from build123d import *

# Parameters (mm, degrees)
SKETCH_R     = 1
SKETCH_W     = 14
SKETCH_H     = 14
PAD_DEPTH    = 1.5
POCKET_START = 1
SKETCH001_R  = 2
POCKET_DEPTH = 14


with BuildPart() as part:
    # Sketch → Pad (new body)
    with BuildSketch(Plane.XY):
        with BuildLine():
            Line((115.15, 33), (115.15, 110.15))
            ThreePointArc((115.15, 110.15), (113.685534, 113.685534), (110.15, 115.15))
            Line((110.15, 115.15), (11, 115.15))
            ThreePointArc((11, 115.15), (7.464466, 113.685534), (6, 110.15))
            Line((6, 110.15), (6, 33))
            ThreePointArc((6, 33), (7.464466, 29.464466), (11, 28))
            Line((11, 28), (110.15, 28))
            ThreePointArc((110.15, 28), (113.685534, 29.464466), (115.15, 33))
        make_face()
        with Locations((10, 111.15)):
            Circle(SKETCH_R, mode=Mode.SUBTRACT)
        with Locations((10, 32)):
            Circle(SKETCH_R, mode=Mode.SUBTRACT)
        with Locations((111.15, 32)):
            Circle(SKETCH_R, mode=Mode.SUBTRACT)
        with Locations((111.15, 111.15)):
            Circle(SKETCH_R, mode=Mode.SUBTRACT)
        with Locations((71.55, 71.55)):
            Circle(SKETCH_R, mode=Mode.SUBTRACT)
        with Locations((33.5, 71.55)):
            Circle(SKETCH_R, mode=Mode.SUBTRACT)
        with Locations((31.5, 62.05)):
            Circle(SKETCH_R, mode=Mode.SUBTRACT)
        with Locations((10, 62.05)):
            Circle(SKETCH_R, mode=Mode.SUBTRACT)
        with Locations((10, 40.55)):
            Circle(SKETCH_R, mode=Mode.SUBTRACT)
        with Locations((31.5, 40.55)):
            Circle(SKETCH_R, mode=Mode.SUBTRACT)
        with Locations((43, 43)):
            Rectangle(SKETCH_W, SKETCH_H, mode=Mode.SUBTRACT)
        with Locations((62.05, 43)):
            Rectangle(SKETCH_W, SKETCH_H, mode=Mode.SUBTRACT)
        with Locations((81.1, 43)):
            Rectangle(SKETCH_W, SKETCH_H, mode=Mode.SUBTRACT)
        with Locations((100.15, 43)):
            Rectangle(SKETCH_W, SKETCH_H, mode=Mode.SUBTRACT)
        with Locations((43, 62.05)):
            Rectangle(SKETCH_W, SKETCH_H, mode=Mode.SUBTRACT)
        with Locations((62.05, 62.05)):
            Rectangle(SKETCH_W, SKETCH_H, mode=Mode.SUBTRACT)
        with Locations((81.1, 62.05)):
            Rectangle(SKETCH_W, SKETCH_H, mode=Mode.SUBTRACT)
        with Locations((100.15, 62.05)):
            Rectangle(SKETCH_W, SKETCH_H, mode=Mode.SUBTRACT)
        with Locations((43, 81.1)):
            Rectangle(SKETCH_W, SKETCH_H, mode=Mode.SUBTRACT)
        with Locations((62.05, 81.1)):
            Rectangle(SKETCH_W, SKETCH_H, mode=Mode.SUBTRACT)
        with Locations((81.1, 81.1)):
            Rectangle(SKETCH_W, SKETCH_H, mode=Mode.SUBTRACT)
        with Locations((100.15, 81.1)):
            Rectangle(SKETCH_W, SKETCH_H, mode=Mode.SUBTRACT)
        with Locations((43, 100.15)):
            Rectangle(SKETCH_W, SKETCH_H, mode=Mode.SUBTRACT)
        with Locations((62.05, 100.15)):
            Rectangle(SKETCH_W, SKETCH_H, mode=Mode.SUBTRACT)
        with Locations((81.1, 100.15)):
            Rectangle(SKETCH_W, SKETCH_H, mode=Mode.SUBTRACT)
        with Locations((100.15, 100.15)):
            Rectangle(SKETCH_W, SKETCH_H, mode=Mode.SUBTRACT)
        with BuildLine():
            ThreePointArc((16.25, 111.15), (15, 112.4), (13.75, 111.15))
            Line((13.75, 111.15), (13.75, 79.15))
            ThreePointArc((13.75, 79.15), (15, 77.9), (16.25, 79.15))
            Line((16.25, 111.15), (16.25, 79.15))
        make_face(mode=Mode.SUBTRACT)
        with BuildLine():
            ThreePointArc((31.25, 111.15), (30, 112.4), (28.75, 111.15))
            Line((28.75, 111.15), (28.75, 79.15))
            ThreePointArc((28.75, 79.15), (30, 77.9), (31.25, 79.15))
            Line((31.25, 111.15), (31.25, 79.15))
        make_face(mode=Mode.SUBTRACT)
        with BuildLine():
            ThreePointArc((15.75, 63.05), (14.75, 62.05), (15.75, 61.05))
            Line((15.75, 61.05), (25.75, 61.05))
            ThreePointArc((25.75, 61.05), (26.75, 62.05), (25.75, 63.05))
            Line((15.75, 63.05), (25.75, 63.05))
        make_face(mode=Mode.SUBTRACT)
    extrude(amount=PAD_DEPTH)

    # Sketch001 → Pocket (cut)
    with BuildSketch(Plane.XY.offset(POCKET_START)):
        with Locations((10, 111.15)):
            Circle(SKETCH001_R)
        with Locations((10, 32)):
            Circle(SKETCH001_R)
        with Locations((111.15, 32)):
            Circle(SKETCH001_R)
        with Locations((111.15, 111.15)):
            Circle(SKETCH001_R)
        with Locations((71.55, 71.55)):
            Circle(SKETCH001_R)
        with Locations((33.5, 71.55)):
            Circle(SKETCH001_R)
    extrude(amount=POCKET_DEPTH, mode=Mode.SUBTRACT)


solid = part.part
The model under review builds one solid part; all positions refer to its coordinate system, in mm. A direction names the side the tool comes from. Coordinates: 2 decimals unless noted, no trailing zeros. Loops run counter-clockwise (first coordinate to the right, second up) from the corner with the lowest first, then second, coordinate; pieces in that order, holes last. Notation, with made-up numbers: (-16.5, 11.5) -> (31.5, 11.5) arc R16 cw to (31.5, 36.5) -> close; hole circle Ø1 at (62.5, -9.5). An arc over 180 degrees is marked (long way). Use a Markdown table: item, result. Add a question column.
1. Add section B-B on z = 0.55. Give the number of separate pieces and of enclosed holes in the cut face, plus the area to 3 significant figures.
2. To check wall thickness, follow line 1 (Y direction, x = 58, z = 1.4); line 2 (X direction, y = 59, z = 0.6); line 3 (X direction, y = 71.55, z = 1.45). State the ranges of each line that lie inside material, in increasing order.
3. Add section A-A on x = 41.5. Write out the cut boundary in (y, z).
4. Machinability: for faces 1 (the face through (35.347, 70.784, 1.246)), 2 (the face through (60, 72, 0)), which of the approach directions +Z, -Z, +X, -X, +Y, -Y give a long, thin tool a straight path to every point of the face, cutting with its end or side? Answer none if there is none.
5. Clearance check with a flat-ended pin moving along its axis: pin 1 Ø2 at (x, y) = (72, 72) entering from +Z. State where the tip first meets the part, or that it passes through.
6. Draft analysis for pull direction X (two halves, no side actions). For faces 3 (the face through (7.5, 113.72, 0.74)), 4 (the face through (60, 72, 1.5)), 5 (the face through (34.4, 70.7, 1)), state which applies: pulls with the +X half, pulls with the -X half, needs draft (parallel to the pull), parting line crosses it, or undercut.
Returned:
| question | item | result |
|---|---|---|
| 1 | separate pieces | 1 |
| 1 | enclosed holes | 29 |
| 1 | area | 6,130 mm² |
| 2 | line 1 | y = 28 to 36, 50 to 55.05, 69.05 to 74.1, 88.1 to 93.15, 107.15 to 115.15 |
| 2 | line 2 | x = 6 to 36, 50 to 55.05, 69.05 to 74.1, 88.1 to 93.15, 107.15 to 115.15 |
| 2 | line 3 | x = 6 to 31.5, 35.5 to 69.55, 73.55 to 115.15 |
| 3 | outline | (28, 0) -> (36, 0) -> (36, 1.5) -> (28, 1.5) -> close; (50, 0) -> (55.05, 0) -> (55.05, 1.5) -> (50, 1.5) -> close; (69.05, 0) -> (74.1, 0) -> (74.1, 1.5) -> (69.05, 1.5) -> close; (88.1, 0) -> (93.15, 0) -> (93.15, 1.5) -> (88.1, 1.5) -> close; (107.15, 0) -> (115.15, 0) -> (115.15, 1.5) -> (107.15, 1.5) -> close |
| 4 | face 1 | +Z |
| 4 | face 2 | -Z, +X, -X, +Y, -Y |
| 5 | pin 1 | stops at z = 1 |
| 6 | face 3 | pulls with the -X half |
| 6 | face 4 | needs draft |
| 6 | face 5 | undercut |
